For this review, use the dimensioned drawing (mm, ordinates from the lowest corner) and the shaded views. Round coordinates to 2 decimals unless told otherwise and drop trailing zeros. Write each loop counter-clockwise with the first axis right and the second up, starting at its lowest first coordinate (ties: lowest second). Pieces come first, ordered by that corner, then holes. Notation, with made-up numbers: M 50.25,-6.5 L 73.25,-6.5 A33 ccw 73.25,27.5 Z; hole C -24.75,-14.75 d3. An arc over 180 degrees is marked long. Use CSV: the item, a comma, the result in double quotes.
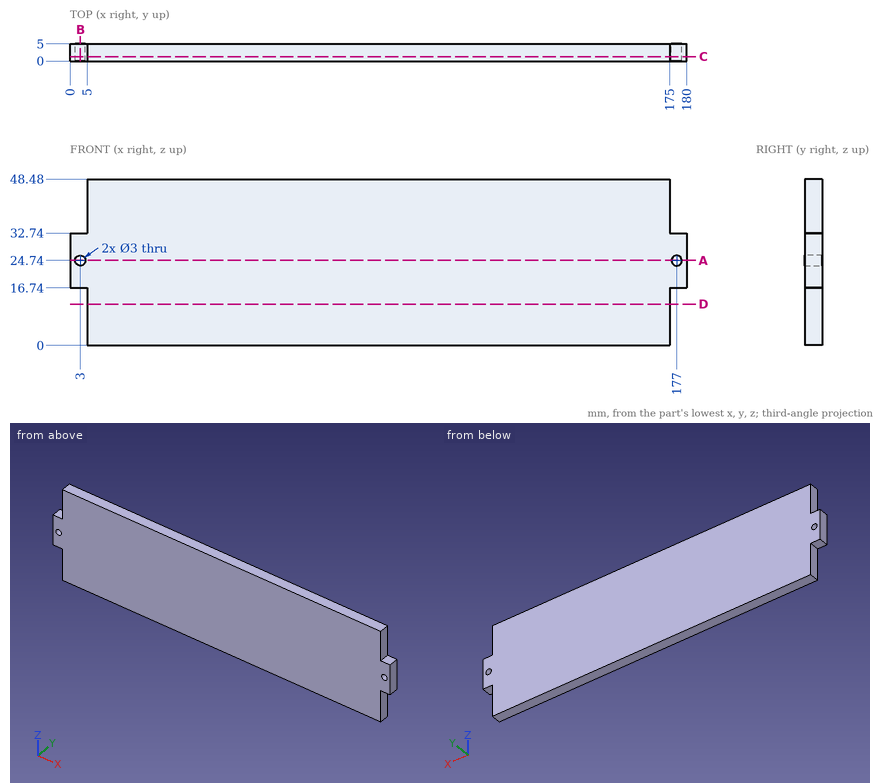
1) Add section D-D on z = 12. Write out the cut boundary in (x, y), then the cut area to 3 significant figures.
Answers:
outline,"M 5,0 L 175,0 L 175,5 L 5,5 Z"
area,"850 mm²"
2) Add section C-C on y = 1.35. Write out the cut boundary in (x, z), then the cut area to 3 significant figures.
Answers:
outline,"M 0,16.74 L 5,16.74 L 5,0 L 175,0 L 175,16.74 L 180,16.74 L 180,32.74 L 175,32.74 L 175,48.48 L 5,48.48 L 5,32.74 L 0,32.74 Z; hole C 3,24.74 d3; hole C 177,24.74 d3"
area,"8,390 mm²"
3) Add section B-B on x = 3. Write out the cut boundary in (y, z), then the cut area to 3 significant figures.
Answers:
outline,"M 0,16.74 L 5,16.74 L 5,23.24 L 0,23.24 Z; M 0,26.24 L 5,26.24 L 5,32.74 L 0,32.74 Z"
area,"65.0 mm²"
4) For pin 1 Ø1.5 at (y, z) = (3, 11.5) entering from +X; pin 2 Ø4 at (x, z) = (3, 24.74) entering from +Y; pin 3 Ø2.5 at (x, y) = (177, 3.5) entering from +Z, all flat-tipped, find the tip position at first contact; note any pin that passes through.
Answers:
pin 1,"x = 175"
pin 2,"y = 5"
pin 3,"z = 32.74"
5) Add section A-A on z = 24.74. Write out the cut boundary in (x, y), then the cut area to 3 significant figures.
Answers:
outline,"M 0,0 L 1.5,0 L 1.5,5 L 0,5 Z; M 4.5,0 L 175.5,0 L 175.5,5 L 4.5,5 Z; M 178.5,0 L 180,0 L 180,5 L 178.5,5 Z"
area,"870 mm²"
6) Wall thickness on line 1 along X through (y, z) = (3.85, 25); line 2 along Z through (x, y) = (3, 1.2); line 3 along X through (y, z) = (3.1, 13): over which ranges is each line inside the solid? List them lowest first. Write a range as [from, to].
Answers:
line 1,"[0, 1.52], [4.48, 175.52], [178.48, 180]"
line 2,"[16.74, 23.24], [26.24, 32.74]"
line 3,"[5, 175]"
